The listing builds one solid part. Answer for the finished solid, in the listing's coordinates (mm). Give positions to 0.01 mm unless a question says otherwise; leave off trailing zeros. Order: outer loops, then holes, each group sorted by start corner. A loop starts at its lowest first (then second) coordinate and runs counter-clockwise, first axis right, second up. Notation, with made-up numbers: (3, -9) - (24, -9) arc R29 ccw to (24, 29) - close; hole circle Ø3 at (49, 5). An arc over 180 degrees is marked (long way). Answer in a Markdown table with one row per item. Add a question column.
```python
from build123d import *

# Parameters (mm, degrees)
SKETCH1_W           = 61
SKETCH1_H           = 1200
BOSS_EXTRUDE1_DEPTH = 12
SKETCH2_R           = 1.25
CUT_EXTRUDE1_DEPTH  = 20
SKETCH3_W           = 23.420452048
SKETCH3_H           = 20
BOSS_EXTRUDE2_DEPTH = 12


with BuildPart() as part:
    # Sketch1 → Boss-Extrude1 (new body)
    with BuildSketch(Plane(origin=(0, 0, 0), x_dir=(1, 0, 0), z_dir=(0, 1, 0))):
        with Locations((30.5, 600)):
            Rectangle(SKETCH1_W, SKETCH1_H)
    extrude(amount=BOSS_EXTRUDE1_DEPTH)

    # Sketch2 → Cut-Extrude1 (cut)
    with BuildSketch(Plane(origin=(0, 12, 0), x_dir=(1, 0, 0), z_dir=(0, 1, 0))):
        with Locations((24.140899916, 77.395)):
            Circle(SKETCH2_R)
        with Locations((24.140899916, 44.395)):
            Circle(SKETCH2_R)
        with Locations((24.140899916, 226.045)):
            Circle(SKETCH2_R)
        with Locations((24.140899916, 193.045)):
            Circle(SKETCH2_R)
        with Locations((24.140899916, 374.695)):
            Circle(SKETCH2_R)
        with Locations((24.140899916, 341.695)):
            Circle(SKETCH2_R)
        with Locations((24.140899916, 523.345)):
            Circle(SKETCH2_R)
        with Locations((24.140899916, 490.345)):
            Circle(SKETCH2_R)
        with Locations((24.140899916, 671.995)):
            Circle(SKETCH2_R)
        with Locations((24.140899916, 638.995)):
            Circle(SKETCH2_R)
        with Locations((24.140899916, 820.645)):
            Circle(SKETCH2_R)
        with Locations((24.140899916, 787.645)):
            Circle(SKETCH2_R)
        with Locations((24.140899916, 969.295)):
            Circle(SKETCH2_R)
        with Locations((24.140899916, 936.295)):
            Circle(SKETCH2_R)
        with Locations((24.140899916, 1117.945)):
            Circle(SKETCH2_R)
        with Locations((24.140899916, 1084.945)):
            Circle(SKETCH2_R)
    extrude(amount=-CUT_EXTRUDE1_DEPTH, mode=Mode.SUBTRACT)

    # Sketch3 → Boss-Extrude2 (add)
    with BuildSketch(Plane(origin=(0, 12, 0), x_dir=(1, 0, 0), z_dir=(0, 1, 0))):
        with Locations((61.289773976, 79.7)):
            Rectangle(SKETCH3_W, SKETCH3_H)
        with Locations((61.289773976, 1120.95)):
            Rectangle(SKETCH3_W, SKETCH3_H)
    extrude(amount=-BOSS_EXTRUDE2_DEPTH)


solid = part.part
```
(1) Find section B-B, the plane z = -723.5. Write down the section's boundary in (x, y).
(2) Find section A-A, the plane y = 8. Give the number of separate pieces and of enclosed holes in the cut face, plus the area to 3 significant figures.
(3) Straight lines are drawn through the part: line 1 (Z direction, x = 70, y = 9.25); line 2 (X direction, y = 6.75, z = -723). For each, find the intervals that lie inside material, in ascending order.
(4) Each of these flat-tipped pins is pushed along its axis until it touches: P1, Ø3.5, axis at y = 8, z = -785.5, coming from the +X side; P2, Ø6, axis at x = 65.5, y = 8.5, coming from the -Z side. Where does it stop, or does it pass through?
Answer key:
| question | item | result |
|---|---|---|
| 1 | outline | (0, 0) - (61, 0) - (61, 12) - (0, 12) - close |
| 2 | separate pieces | 1 |
| 2 | enclosed holes | 16 |
| 2 | area | 73,600 mm² |
| 3 | line 1 | -1130.95 to -1110.95, -89.7 to -69.7 |
| 3 | line 2 | 0 to 61 |
| 4 | P1 | x = 61 |
| 4 | P2 | z = -1130.95 |
